Read the model definition and answer for the solid it produces. Units are mm, in the model's axes. A direction names the side the tool comes from. Coordinates: 2 decimals unless noted, no trailing zeros. Loops run counter-clockwise (first coordinate to the right, second up) from the corner with the lowest first, then second, coordinate; pieces in that order, holes last. Notation, with made-up numbers: M 84,75 L 99,75 A25 ccw 99,112 Z; hole C -27,18.25 d7. An arc over 180 degrees is marked long. One line per item, written item: value. Start each with the question number.
1. Flat-ended cylindrical pins translate along their axes: pin 1 (8.5 mm diameter, centred on y = -14.5, z = 17, fed in from -X) (3 decimals); pin 2 (1.5 mm diameter, centred on x = 0.5, z = 15.5, fed in from +Y); pin 3 (15.5 mm diameter, centred on x = 18, z = 34, fed in from -Y). Find the tip coordinate at first contact, or state that the pin passes through.
2. Determine the mould class of faces 1 (the face through (60, 2, 42.875)), 2 (the face through (46, 25.4, 42)), 3 (the face through (30.879, -16.791, 50.013)), 4 (the face through (45.8, -0.4, 38.1)) for opening direction X: +X half, -X half, draft (parallel to the pull), parting line (faces both ways), or undercut.
3. The part is cut by section C-C (y = -49). Write down the section's boundary in (x, z) (3 decimals), then the cut area to 3 significant figures.
4. The part is cut by section A-A (x = 71). Write down the section's boundary in (y, z) (3 decimals).
5. For faces 5 (the face through (46, -25.4, 42)), 6 (the face through (60, -2, 61.925)), 7 (the face through (-6, 7.938, 30)), 8 (the face through (22.225, -17, 18)), 9 (the face through (86, 0, 38.1)), determine the directions among +Z, -Z, +X, -X, +Y, -Y from which every point of the face is accessible in a straight line to the end or side of a thin tool.
6. The part is cut by section B-B (z = 6.5). Write down the section's boundary in (x, y) (3 decimals).
7. Consider probe 1 along Z at (x, y) = (15.5, 33.5) (3 decimals); probe 2 along X at (y, z) = (11, 16) (3 decimals); probe 3 along X at (y, z) = (43, -4.5) (3 decimals). Determine where each line is inside the solid, lowest interval first.
```python
from build123d import *

# Parameters (mm, degrees)
F1_DEPTH = 63.5
F2_DEPTH = 7.9375
F0_W     = 25.4
F0_H     = 19.05
F3_DEPTH = 25.4


with BuildPart() as f1:
    # F0 (on Front) → F1 (new body, symmetric)
    with BuildSketch(Plane.XZ):
        Polygon((41.275, -9.525), (41.275, 9.525), (22.225, 9.525), (-41.275, 9.525), (-41.275, -9.525), align=None)
    extrude(amount=F1_DEPTH, both=True)

    # F0 (on Front) → F2 (join, symmetric)
    with BuildSketch(Plane.XZ):
        with BuildLine():
            Line((-41.275, 9.525), (22.225, 9.525))
            Line((22.225, 9.525), (22.225, 27.0002))
            ThreePointArc((22.225, 27.0002), (30.6519829848, 49.7512597394), (51.8662723988, 61.5232046148))
            add(Edge.make_bspline(
                [(-41.275, 9.525), (-42.4839697901, 38.0803204512), (17.0147305919, 58.0960971438), (51.8662723988, 61.5232046148)],
                knots=[0, 0, 0, 0, 105.9312779521, 105.9312779521, 105.9312779521, 105.9312779521], degree=3))
        make_face()
    extrude(amount=F2_DEPTH, both=True)

    # F0 (on Front) → F3 (join, symmetric)
    with BuildSketch(Plane.XZ):
        with BuildLine():
            Line((22.225, 9.525), (41.275, 9.525))
            Line((41.275, 9.525), (41.275, 27.0002))
            ThreePointArc((41.275, 27.0002), (45.9246798487, 38.2255201513), (57.15, 42.8752))
            Line((57.15, 42.8752), (60.325, 42.8752))
            Line((60.325, 42.8752), (60.325, 61.9252))
            Line((60.325, 61.9252), (57.15, 61.9252))
            add(Edge.make_bspline(
                [(51.8662723988, 61.5232046148), (53.6998823137, 61.7035116518), (55.4652682936, 61.8379008486), (57.15, 61.9252)],
                knots=[105.9312779521, 105.9312779521, 105.9312779521, 105.9312779521, 111.5045361635, 111.5045361635, 111.5045361635, 111.5045361635], degree=3))
            ThreePointArc((51.8662723988, 61.5232046148), (30.6519829848, 49.7512597394), (22.225, 27.0002))
            Line((22.225, 27.0002), (22.225, 9.525))
        make_face()
        with Locations((73.025, 52.4002)):
            Rectangle(F0_W, F0_H)
    extrude(amount=F3_DEPTH, both=True)

    # F0 (on Front) → F4 (revolve)
    with BuildSketch(Plane.XZ):
        Polygon((85.725, 61.9252), (85.725, 42.8752), (85.725, 38.1), (111.125, 38.1), (111.125, 66.675), (85.725, 66.675), align=None)
    revolve(axis=Axis((85.725, 0, 52.3875), (0, 0, -1)))


solid = f1.part
```
Answer block:
1. pin 1: stops at x = 22.225
1. pin 2: stops at y = 7.94
1. pin 3: stops at y = -25.4
2. face 1: undercut
2. face 2: draft
2. face 3: -X half
2. face 4: undercut
3. outline: M -41.275,-9.525 L 41.275,-9.525 L 41.275,9.525 L -41.275,9.525 Z
3. area: 1,570 mm2
4. outline: M -25.4,42.875 L -20.696,42.875 L -20.696,38.1 L 20.696,38.1 L 20.696,42.875 L 25.4,42.875 L 25.4,61.925 L 20.696,61.925 L 20.696,66.675 L -20.696,66.675 L -20.696,61.925 L -25.4,61.925 Z
5. face 5: +Z, +X, -X, -Y
5. face 6: +Z, -X
5. face 7: +Z, -X, +Y
5. face 8: +Z, -X, -Y
5. face 9: -Z, +X, +Y, -Y
6. outline: M -41.275,-63.5 L 41.275,-63.5 L 41.275,63.5 L -41.275,63.5 Z
7. probe 1: z = -9.525 to 9.525
7. probe 2: x = 22.225 to 41.275
7. probe 3: x = -41.275 to 41.275
